The listing builds one solid part. Answer for the finished solid, in the listing's coordinates (mm). A direction names the side the tool comes from. Round coordinates to 2 decimals unless told otherwise and drop trailing zeros. Write each loop counter-clockwise with the first axis right and the second up, starting at its lowest first coordinate (ties: lowest second). Pieces come first, ordered by that corner, then holes.
Item 1: Find section A-A on z = 0. Give the vertices of the cut face in (x, y).
Item 2: A tool of negligible diameter and unlimited length cuts with its end or side. For faces 4 (the face through (-10, 49, -7)), 5 (the face through (5.08, 49.3, 6.14)), 6 (the face through (4, 49, 0)), from which of +Z, -Z, +X, -X, +Y, -Y can it reach the whole face along a straight path? Write none if from no direction.
Item 3: Find the intervals of material crossed by probe 1 along X at (y, z) = (69.5, 8.75); probe 2 along X at (y, z) = (23, 0), in increasing order.
Item 4: For a pull along Z with two mould halves and no side action, classify faces 1 (the face through (10, 49, -7)), 2 (the face through (0, 49, 4)), 3 (the face through (8.5, 49, -5)) as +Z half, -Z half, draft (parallel to the pull), parting line (faces both ways), or undercut.
Item 5: Each of these flat-tipped pins is pushed along its axis until it touches: pin 1 (3.5 mm diameter, centred on y = 49, z = -0.5, fed in from +X); pin 2 (1 mm diameter, centred on x = 4, z = -7, fed in from -Y). Where does it stop, or does it pass through?
Item 6: Find section B-B on x = 0. Give the vertices of the cut face in (y, z), then the cut area to 3 significant figures.
```python
from build123d import *

# Parameters (mm, degrees)
SKETCH1_R           = 2.5
BOSS_EXTRUDE1_DEPTH = 100


with BuildPart() as part:
    # Sketch1 → Boss-Extrude1 (new body)
    with BuildSketch(Plane(origin=(0, 0, 0), x_dir=(1, 0, 0), z_dir=(0, 1, 0))):
        with BuildLine():
            Line((-3.610984523, 4.671644695), (-6.585786438, 7.646446609))
            ThreePointArc((-6.585786438, 7.646446609), (-6.694172813, 8.191341716), (-6.232233047, 8.5))
            Line((-6.232233047, 8.5), (-4.2, 8.5))
            Line((-4.2, 8.5), (-4.2, 10))
            Line((-4.2, 10), (-9.25, 10))
            ThreePointArc((-9.25, 10), (-9.780330086, 9.780330086), (-10, 9.25))
            Line((-10, 9.25), (-10, 4.2))
            Line((-10, 4.2), (-8.5, 4.2))
            Line((-8.5, 4.2), (-8.5, 6.232233047))
            ThreePointArc((-8.5, 6.232233047), (-8.191341716, 6.694172813), (-7.646446609, 6.585786438))
            Line((-7.646446609, 6.585786438), (-4.671644695, 3.610984523))
            ThreePointArc((-4.671644695, 3.610984523), (-4.244383234, 2.985253206), (-4, 2.268058063))
            Line((-4, 2.268058063), (-4, -2.268058063))
            ThreePointArc((-4, -2.268058063), (-4.244383234, -2.985253206), (-4.671644695, -3.610984523))
            Line((-4.671644695, -3.610984523), (-7.646446609, -6.585786438))
            ThreePointArc((-7.646446609, -6.585786438), (-8.191341716, -6.694172813), (-8.5, -6.232233047))
            Line((-8.5, -6.232233047), (-8.5, -4.2))
            Line((-8.5, -4.2), (-10, -4.2))
            Line((-10, -4.2), (-10, -9.25))
            ThreePointArc((-10, -9.25), (-9.780330086, -9.780330086), (-9.25, -10))
            Line((-9.25, -10), (-4.2, -10))
            Line((-4.2, -10), (-4.2, -8.5))
            Line((-4.2, -8.5), (-6.232233047, -8.5))
            ThreePointArc((-6.232233047, -8.5), (-6.694172813, -8.191341716), (-6.585786438, -7.646446609))
            Line((-6.585786438, -7.646446609), (-3.610984523, -4.671644695))
            ThreePointArc((-3.610984523, -4.671644695), (-2.985253206, -4.244383234), (-2.268058063, -4))
            Line((-2.268058063, -4), (2.268058063, -4))
            ThreePointArc((2.268058063, -4), (2.985253206, -4.244383234), (3.610984523, -4.671644695))
            Line((3.610984523, -4.671644695), (6.585786438, -7.646446609))
            ThreePointArc((6.585786438, -7.646446609), (6.694172813, -8.191341716), (6.232233047, -8.5))
            Line((6.232233047, -8.5), (4.2, -8.5))
            Line((4.2, -8.5), (4.2, -10))
            Line((4.2, -10), (9.25, -10))
            ThreePointArc((9.25, -10), (9.780330086, -9.780330086), (10, -9.25))
            Line((10, -9.25), (10, -4.2))
            Line((10, -4.2), (8.5, -4.2))
            Line((8.5, -4.2), (8.5, -6.232233047))
            ThreePointArc((8.5, -6.232233047), (8.191341716, -6.694172813), (7.646446609, -6.585786438))
            Line((7.646446609, -6.585786438), (4.671644695, -3.610984523))
            ThreePointArc((4.671644695, -3.610984523), (4.244383234, -2.985253206), (4, -2.268058063))
            Line((4, -2.268058063), (4, 2.268058063))
            ThreePointArc((4, 2.268058063), (4.244383234, 2.985253206), (4.671644695, 3.610984523))
            Line((4.671644695, 3.610984523), (7.646446609, 6.585786438))
            ThreePointArc((7.646446609, 6.585786438), (8.191341716, 6.694172813), (8.5, 6.232233047))
            Line((8.5, 6.232233047), (8.5, 4.2))
            Line((8.5, 4.2), (10, 4.2))
            Line((10, 4.2), (10, 9.25))
            ThreePointArc((10, 9.25), (9.780330086, 9.780330086), (9.25, 10))
            Line((9.25, 10), (4.2, 10))
            Line((4.2, 10), (4.2, 8.5))
            Line((4.2, 8.5), (6.232233047, 8.5))
            ThreePointArc((6.232233047, 8.5), (6.694172813, 8.191341716), (6.585786438, 7.646446609))
            Line((6.585786438, 7.646446609), (3.610984523, 4.671644695))
            ThreePointArc((3.610984523, 4.671644695), (2.985253206, 4.244383234), (2.268058063, 4))
            Line((2.268058063, 4), (-2.268058063, 4))
            ThreePointArc((-2.268058063, 4), (-2.985253206, 4.244383234), (-3.610984523, 4.671644695))
        make_face()
        Circle(SKETCH1_R, mode=Mode.SUBTRACT)
    extrude(amount=BOSS_EXTRUDE1_DEPTH)


solid = part.part
```
Check values:
1. outline: (-4, 0) - (-2.5, 0) - (-2.5, 100) - (-4, 100) - close; (2.5, 0) - (4, 0) - (4, 100) - (2.5, 100) - close
2. face 4: +Z, -Z, -X, +Y, -Y
2. face 5: +Y, -Y
2. face 6: +X, +Y, -Y
3. probe 1: x = -10 to -4.2, 4.2 to 10
3. probe 2: x = -4 to -2.5, 2.5 to 4
4. face 1: draft
4. face 2: +Z half
4. face 3: undercut
5. pin 1: stops at x = 4
5. pin 2: passes through
6. outline: (0, -4) - (100, -4) - (100, -2.5) - (0, -2.5) - close; (0, 2.5) - (100, 2.5) - (100, 4) - (0, 4) - close
6. area: 300 mm2
